```python
from build123d import *

# Parameters (mm, degrees)
BOSS_EXTRUDE1_DEPTH = 3.175
SKETCH2_R           = 5.715
BOSS_EXTRUDE2_DEPTH = 0.8128


with BuildPart() as part:
    # Sketch1 → Boss-Extrude1 (new body)
    with BuildSketch(Plane.XY):
        Polygon((3.666174209, 0), (1.833087105, 3.175), (-1.833087105, 3.175), (-3.666174209, 0), (-1.833087105, -3.175), (1.833087105, -3.175), align=None)
    extrude(amount=BOSS_EXTRUDE1_DEPTH)

    # Sketch2 → Boss-Extrude2 (add)
    with BuildSketch(Plane.XY.offset(3.175)):
        Circle(SKETCH2_R)
    extrude(amount=BOSS_EXTRUDE2_DEPTH)

    # Sketch3 → Revolve1 (revolve)
    with BuildSketch(Plane(origin=(0, 0, 0), x_dir=(0, 0, -1), z_dir=(1, 0, 0)), mode=Mode.PRIVATE) as revolve1_sk:
        Polygon((-3.9878, 0), (-49.4378, 0), (-49.4378, 2.145), (-39.3678, 2.145), (-39.3678, 1), (-38.3678, 1), (-38.3678, 2.145), (-3.9878, 2.145), align=None)
    revolve(revolve1_sk.sketch.rotate(Axis((0, 0, 3.9878), (0, 0, 1)), 90), axis=Axis((0, 0, 3.9878), (0, 0, 1)))


solid = part.part
```
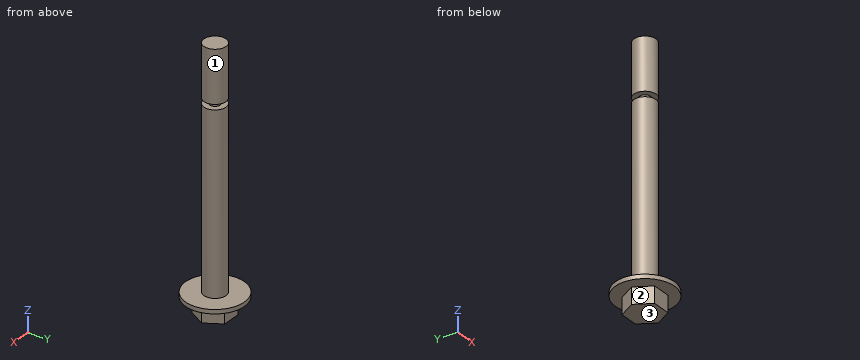
CAD build for the part. Positions are in the model's coordinates, mm. Face numbers are marked on the shaded views. A direction names the side the tool comes from. Give positions to 0.01 mm unless a question says otherwise; leave off trailing zeros. Write each loop counter-clockwise with the first axis right and the second up, starting at its lowest first coordinate (ties: lowest second). Pieces come first, ordered by that corner, then holes. Notation, with made-up numbers: M 32.5,-7 L 60.5,-7 A17 cw 60.5,4 Z; hole C 15,-33.75 d10. An arc over 180 degrees is marked long. Return JSON: item names as keys, results as strings. Group by question number.
(1) Band-saw the part on C-C (z = 7.5). Give the cut face in (x, y) (3 decimals).
(2) Band-saw the part on D-D (y = -4.25). Give the cut face in (x, z) (3 decimals), and give its area (3 significant figures).
(3) Flat gauge pins, fed straight in: pin 1 Ø4 at (x, z) = (-0.5, 21.5) entering from -Y (3 decimals); pin 2 Ø2 at (y, z) = (-4.5, 20.5) entering from -X; pin 3 Ø3 at (y, z) = (0.5, 42.5) entering from +X (3 decimals); pin 4 Ø1 at (x, z) = (0.5, 2) entering from +Y (3 decimals). Where does each tip first touch, or does it go through?
(4) Band-saw the part on B-B (y = -0.5). Give the cut face in (x, z) (1 decimal), and give its area (3 significant figures).
(5) Drill centre lines: L1, parallel to Z at x = 1.25, y = 1.25; L2, parallel to Z at x = -3.75, y = 0.25 (3 decimals); L3, parallel to Z at x = -0.75, y = 3. Where is each one in solid material? Low to high. Write a range as [from, to].
(6) Band-saw the part on A-A (x = 0). Give the cut face in (y, z) (3 decimals), and give its area (3 significant figures).
(7) 3-axis set-ups, long thin cutter, end or side, ignore diameter. For the marked faces 1, 2 and 3: which of +Z, -Z, +X, -X, +Y, -Y reach the whole face in a straight line?
Entries:
{
 "1": {"outline": "C 0,0 d4.29"},
 "2": {"outline": "M -3.821,3.175 L 3.821,3.175 L 3.821,3.988 L -3.821,3.988 Z", "area": "6.21 mm^2"},
 "3": {"pin 1": "stops at y = -2.145", "pin 2": "passes through", "pin 3": "stops at x = 2.145", "pin 4": "stops at y = 3.175"},
 "4": {"outline": "M -5.7,3.2 L -3.4,3.2 L -3.4,0 L 3.4,0 L 3.4,3.2 L 5.7,3.2 L 5.7,4 L 2.1,4 L 2.1,38.4 L 0.9,38.4 L 0.9,39.4 L 2.1,39.4 L 2.1,49.4 L -2.1,49.4 L -2.1,39.4 L -0.9,39.4 L -0.9,38.4 L -2.1,38.4 L -2.1,4 L -5.7,4 Z", "area": "218 mm^2"},
 "5": {"L1": "z = [0, 38.37], [39.37, 49.44]", "L2": "z = [3.175, 3.988]", "L3": "z = [0, 3.99]"},
 "6": {"outline": "M -5.715,3.175 L -3.175,3.175 L -3.175,0 L 3.175,0 L 3.175,3.175 L 5.715,3.175 L 5.715,3.988 L 2.145,3.988 L 2.145,38.368 L 1,38.368 L 1,39.368 L 2.145,39.368 L 2.145,49.438 L -2.145,49.438 L -2.145,39.368 L -1,39.368 L -1,38.368 L -2.145,38.368 L -2.145,3.988 L -5.715,3.988 Z", "area": "222 mm^2"},
 "7": {"face 1": "+Z", "face 2": "-Z, -X, -Y", "face 3": "-Z, +X, -X, +Y, -Y"}
}
